The listing builds one solid part. Answer for the finished solid, in the listing's coordinates (mm). A direction names the side the tool comes from. Round coordinates to 2 decimals unless told otherwise and drop trailing zeros. Write each loop counter-clockwise with the first axis right and the second up, starting at its lowest first coordinate (ties: lowest second). Pieces come first, ordered by that corner, then holes. Notation, with made-up numbers: (54.25, 45.5) - (85.25, 45.5) arc R10 ccw to (85.25, 55.5) - close; hole circle Ø2 at (33.5, 80). An arc over 180 degrees is marked (long way). Use a Markdown table: item, result. Add a question column.
1) A cutting plane is placed at B-B (z = 17.25). Give the vertices of the cut face in (x, y).
2) Find the intervals of material crossed by probe 1 along X at (y, z) = (-10, -2.45); probe 2 along Y at (x, z) = (-15, -2.7); probe 3 along X at (y, z) = (-8.75, 2), in increasing order. Write a range as from..to.
3) A cutting plane is placed at A-A (x = -6). Give the vertices of the cut face in (y, z).
4) A cutting plane is placed at D-D (y = -4). Give the vertices of the cut face in (x, z), then the cut area to 3 significant figures.
5) Each of these flat-tipped pins is pushed along its axis until it touches: P1, Ø10, axis at y = -6.5, z = 10, coming from the +X side; P2, Ø6, axis at x = 15, y = -10, coming from the +Z side; P3, Ø2, axis at x = 15.5, z = 1.5, coming from the +Y side; P4, Ø11, axis at x = -17, y = -6, coming from the +Z side. Where does it stop, or does it pass through?
6) A cutting plane is placed at C-C (y = -18.5). Give the vertices of the cut face in (x, z).
7) Determine the mould class of faces 4 (the conical face through (-14.69, -7.66, -2.12)), 5 (the conical face through (16.738, -8.406, -2.122)), 6 (the flat face through (-15, -5, 0)), 7 (the flat face through (-0.14, -15.07, 11.34)) for opening direction Y: +Y half, -Y half, draft (parallel to the pull), parting line (faces both ways), or undercut.
8) A tool of negligible diameter and unlimited length cuts with its end or side. For faces 1 (the flat face through (10, -8, 11)), 2 (the cylindrical face through (13.79, -8.103, -2.62)), 3 (the flat face through (-10, -8, 11)), from which of +Z, -Z, +X, -X, +Y, -Y can it reach the whole face along a straight path? Write none if from no direction.
```python
from build123d import *

# Parameters (mm, degrees)
F0_W           = 20
F0_H           = 23
F1_DEPTH       = 20
F2_SIZE2       = 23
F2_SIZE        = 10
F4_D           = 4.5
F4_DEPTH       = 12
F4_CSINK_D     = 8.96
F4_CSINK_ANGLE = 90
F4_TIP         = 1.3519363928
F5_R           = 5


with BuildPart() as f1:
    # F0 (on Front) → F1 (new body)
    with BuildSketch(Plane.XZ):
        with Locations((0, 11.5)):
            Rectangle(F0_W, F0_H)
        Polygon((10, 0), (-10, 0), (-20, 0), (-20, -3), (20, -3), (20, 0), align=None)
    extrude(amount=F1_DEPTH)

    # F2
    f2_edges = [f1.edges().sort_by_distance(p)[0] for p in [
        (0, -20, 23),
    ]]
    f2_side = f1.faces().sort_by_distance((0, -10, 23))[0]
    chamfer(f2_edges, length=F2_SIZE, length2=F2_SIZE2, reference=f2_side)

    # F4
    with Locations(Plane.XY):
        with Locations((-15, -10), (15, -10)):
            CounterSinkHole(F4_D / 2, F4_CSINK_D / 2, depth=F4_DEPTH, counter_sink_angle=F4_CSINK_ANGLE)
            with Locations((0, 0, -(F4_DEPTH + F4_TIP / 2))):  # 118° drill point
                Cone(0, F4_D / 2, F4_TIP, mode=Mode.SUBTRACT)

    # F5
    f5_edges = [f1.edges().sort_by_distance(p)[0] for p in [
        (-20, -20, -1.5),
        (20, -20, -1.5),
        (-20, 0, -1.5),
        (20, 0, -1.5),
    ]]
    fillet(f5_edges, radius=F5_R)


solid = f1.part
```
Entries:
| question | item | result |
|---|---|---|
| 1 | outline | (-10, -12.5) - (10, -12.5) - (10, 0) - (-10, 0) - close |
| 2 | probe 1 | x = -20..-17.25, -12.75..12.75, 17.25..20 |
| 2 | probe 2 | y = -20..-12.25, -7.75..0 |
| 2 | probe 3 | x = -10..10 |
| 3 | outline | (-20, -3) - (0, -3) - (0, 23) - (-10, 23) - (-20, 0) - close |
| 4 | outline | (-19.9, -3) - (19.9, -3) - (19.9, 0) - (10, 0) - (10, 23) - (-10, 23) - (-10, 0) - (-19.9, 0) - close |
| 4 | area | 579 mm² |
| 5 | P1 | stops at x = 10 |
| 5 | P2 | stops at z = -1.48 |
| 5 | P3 | passes through |
| 5 | P4 | stops at z = 0 |
| 6 | outline | (-18.57, -3) - (18.57, -3) - (18.57, 0) - (10, 0) - (10, 3.45) - (-10, 3.45) - (-10, 0) - (-18.57, 0) - close |
| 7 | face 4 | undercut |
| 7 | face 5 | undercut |
| 7 | face 6 | draft |
| 7 | face 7 | -Y half |
| 8 | face 1 | +Z, +X, +Y, -Y |
| 8 | face 2 | +Z, -Z |
| 8 | face 3 | +Z, -X, +Y, -Y |
